Geometry check sheet. Reference: drawing and pictorial views, mm from the part's lowest x, y, z. A direction names the side the tool comes from. Round coordinates to 2 decimals unless told otherwise and drop trailing zeros. Write each loop counter-clockwise with the first axis right and the second up, starting at its lowest first coordinate (ties: lowest second). Pieces come first, ordered by that corner, then holes. Notation, with made-up numbers: (57, -34) -> (104, -34) arc R24 cw to (104, -15) -> close; hole circle Ø4 at (-35, -12). An arc over 180 degrees is marked (long way). Answer as a JSON object with one key per item and string values. Group by question number.
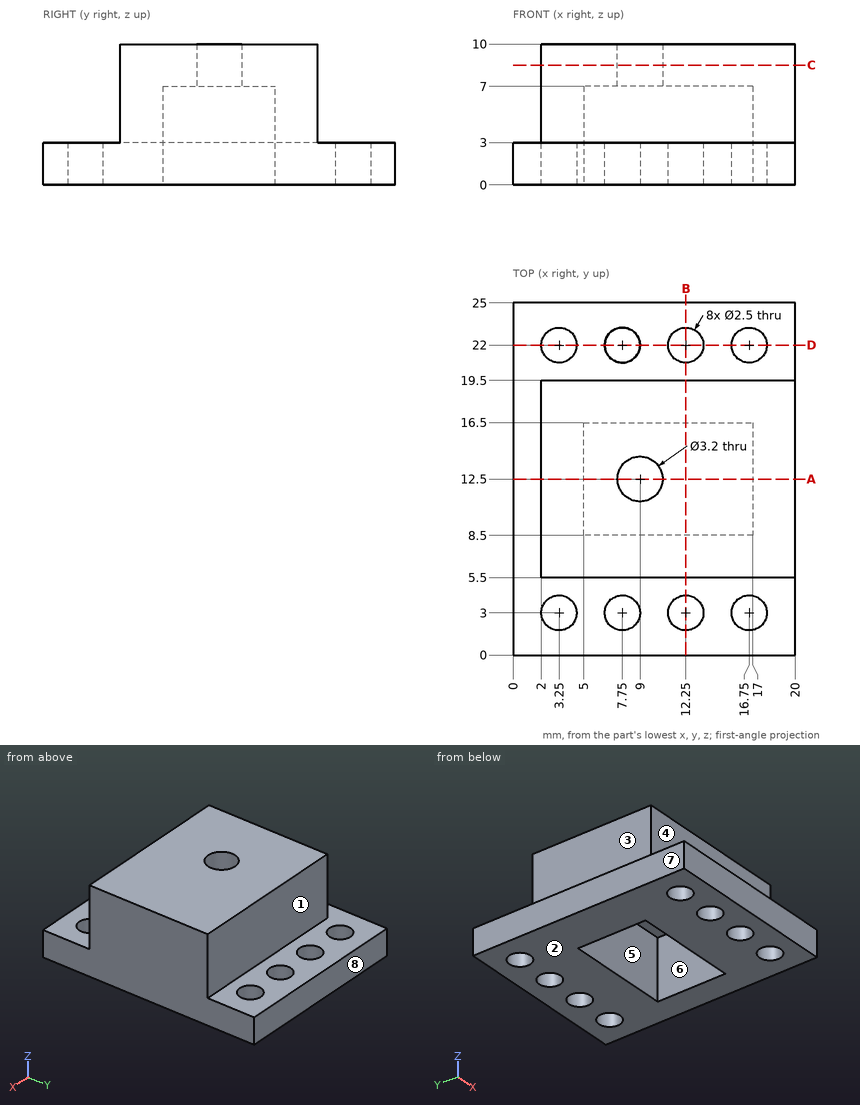
(1) Section check C-C on z = 8.5. Record the cut outline in (x, y).
(2) Section check D-D on y = 22. Record the cut outline in (x, z).
(3) Section check A-A on y = 12.5. Record the cut outline in (x, z), then the cut area to 3 significant figures.
(4) Section check B-B on x = 12.25. Record the cut outline in (y, z), then the cut area to 3 significant figures.
(5) Scan lines: line 1 along Y through (x, z) = (7.75, 1.8); line 2 along X through (y, z) = (12.75, 5.25); line 3 along Y through (x, z) = (3.25, 2.1). Record each from-to range of solid material in increasing order.
(6) Release check for a two-part mould opening along Y. For the marked faces 6, 7 and 8 record: pulls with the +Y half, pulls with the -Y half, needs draft (parallel to the pull), parting line crosses it, or undercut.
(7) Go/stop test with flat-tipped pins: pin 1 Ø6.5 at (x, y) = (13, 14.5) entering from -Z; pin 2 Ø3 at (x, y) = (16.75, 3) entering from +Z; pin 3 Ø2 at (x, z) = (12, 4.5) entering from -Y; pin 4 Ø2 at (y, z) = (12, 6.5) entering from -X. Record where each tip stops, or that it passes through.
(8) Access from +Z, -Z, +X, -X, +Y, -Y to the whole of each face (thin tool, end or side, straight path). Record for the marked faces 1, 2, 3, 4 and 5.
Data:
{
 "1": {"outline": "(2, 5.5) -> (20, 5.5) -> (20, 19.5) -> (2, 19.5) -> close; hole circle Ø3.2 at (9, 12.5)"},
 "2": {"outline": "(0, 0) -> (2, 0) -> (2, 3) -> (0, 3) -> close; (4.5, 0) -> (6.5, 0) -> (6.5, 3) -> (4.5, 3) -> close; (9, 0) -> (11, 0) -> (11, 3) -> (9, 3) -> close; (13.5, 0) -> (15.5, 0) -> (15.5, 3) -> (13.5, 3) -> close; (18, 0) -> (20, 0) -> (20, 3) -> (18, 3) -> close"},
 "3": {"outline": "(0, 0) -> (5, 0) -> (5, 7) -> (7.4, 7) -> (7.4, 10) -> (2, 10) -> (2, 3) -> (0, 3) -> close; (10.6, 7) -> (17, 7) -> (17, 0) -> (20, 0) -> (20, 10) -> (10.6, 10) -> close", "area": "92.4 mm²"},
 "4": {"outline": "(0, 0) -> (1.75, 0) -> (1.75, 3) -> (0, 3) -> close; (4.25, 0) -> (8.5, 0) -> (8.5, 7) -> (16.5, 7) -> (16.5, 0) -> (20.75, 0) -> (20.75, 3) -> (19.5, 3) -> (19.5, 10) -> (5.5, 10) -> (5.5, 3) -> (4.25, 3) -> close; (23.25, 0) -> (25, 0) -> (25, 3) -> (23.25, 3) -> close", "area": "102 mm²"},
 "5": {"line 1": "y = 0 to 1.75, 4.25 to 8.5, 16.5 to 20.75, 23.25 to 25", "line 2": "x = 2 to 5, 17 to 20", "line 3": "y = 0 to 1.75, 4.25 to 20.75, 23.25 to 25"},
 "6": {"face 6": "undercut", "face 7": "needs draft", "face 8": "pulls with the +Y half"},
 "7": {"pin 1": "stops at z = 0", "pin 2": "stops at z = 3", "pin 3": "stops at y = 5.5", "pin 4": "stops at x = 2"},
 "8": {"face 1": "+Z, +X, -X, +Y", "face 2": "-Z, +X, -X, +Y, -Y", "face 3": "+Z, -X, +Y, -Y", "face 4": "+Z, +X, -X, -Y", "face 5": "-Z"}
}
